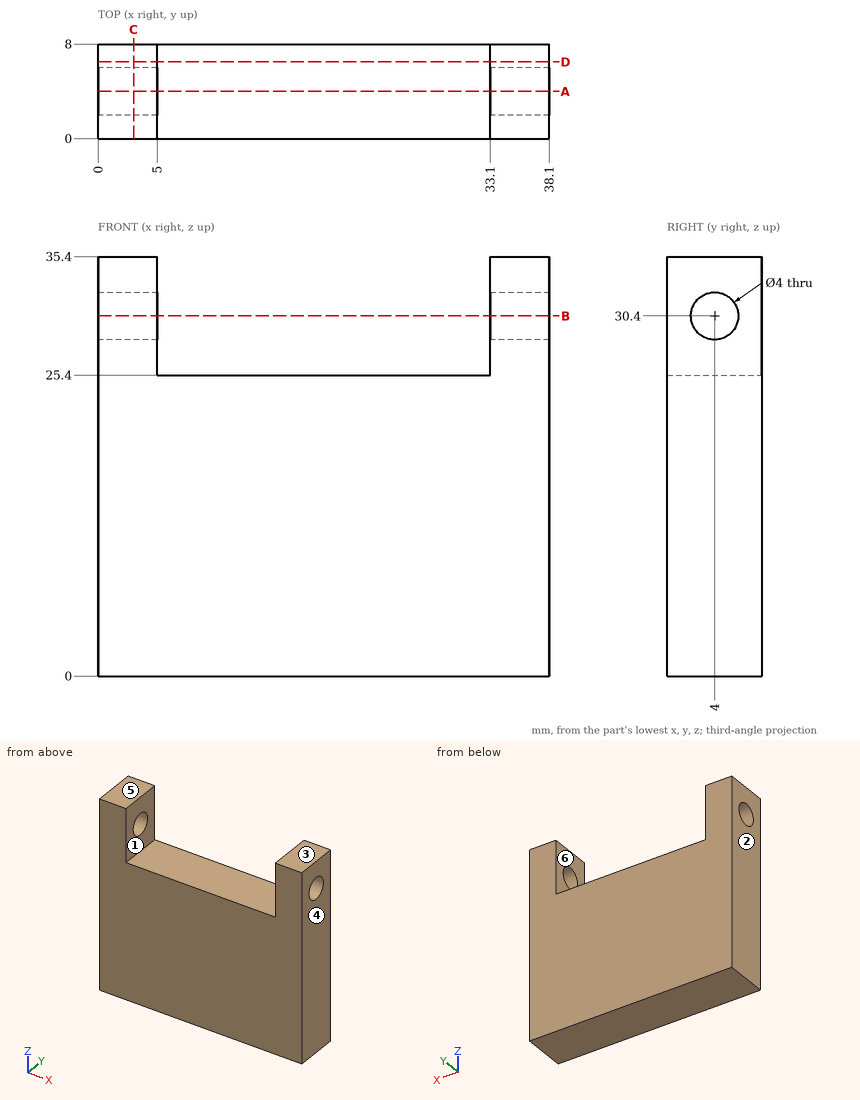
Verification items for this drawing (mm, ordinates from the low corner). A direction names the side the tool comes from. Round coordinates to 2 decimals unless told otherwise and drop trailing zeros. Order: outer loops, then holes, each group sorted by start corner. A loop starts at its lowest first (then second) coordinate and runs counter-clockwise, first axis right, second up.
1) Material ranges on line 1 (X direction, y = 6.5, z = 29); line 2 (Y direction, x = 35.3, z = 30.4); line 3 (Z direction, x = 20, y = 1.25), recorded low to high.
Geometry says:
line 1: x = 0 to 5, 33.1 to 38.1
line 2: y = 0 to 2, 6 to 8
line 3: z = 0 to 25.4
2) Cross-section at A-A, the plane y = 4. Record the cut outline in (x, z).
Geometry says:
outline: (0, 0) - (38.1, 0) - (38.1, 28.4) - (33.1, 28.4) - (33.1, 25.4) - (5, 25.4) - (5, 28.4) - (0, 28.4) - close; (0, 32.4) - (5, 32.4) - (5, 35.4) - (0, 35.4) - close; (33.1, 32.4) - (38.1, 32.4) - (38.1, 35.4) - (33.1, 35.4) - close
3) Tool access check on the marked faces 5 and 6. Record the directions out of +Z, -Z, +X, -X, +Y, -Y that give a thin tool (end or side, any length) a straight path to the whole face; none if there is none.
Geometry says:
face 5: +Z, +X, -X, +Y, -Y
face 6: +Z, +Y, -Y
4) Draft check along X on the marked faces 1, 2, 3 and 4. Enter one of: +X half, -X half, draft (parallel to the pull), parting line (faces both ways), or undercut.
Geometry says:
face 1: undercut
face 2: -X half
face 3: draft
face 4: +X half
5) Cross-section at D-D, the plane y = 6.5. Record the cut outline in (x, z), plus the area to 3 significant figures.
Geometry says:
outline: (0, 0) - (38.1, 0) - (38.1, 35.4) - (33.1, 35.4) - (33.1, 25.4) - (5, 25.4) - (5, 35.4) - (0, 35.4) - close
area: 1,070 mm2
6) Depth check by flat-ended pin: pin 1 (2.5 mm diameter, centred on x = 13, y = 5, fed in from +Z). Enter the tip coordinate at first touch or a pass-through.
Geometry says:
pin 1: stops at z = 25.4
7) Cross-section at B-B, the plane z = 30.4. Record the cut outline in (x, y).
Geometry says:
outline: (0, 0) - (5, 0) - (5, 2) - (0, 2) - close; (0, 6) - (5, 6) - (5, 8) - (0, 8) - close; (33.1, 0) - (38.1, 0) - (38.1, 2) - (33.1, 2) - close; (33.1, 6) - (38.1, 6) - (38.1, 8) - (33.1, 8) - close
8) Cross-section at C-C, the plane x = 3. Record the cut outline in (y, z).
Geometry says:
outline: (0, 0) - (8, 0) - (8, 35.4) - (0, 35.4) - close; hole circle Ø4 at (4, 30.4)
